from build123d import *

# Parameters (mm, degrees)
SKETCH_1_R      = 1.5
SKETCH_1_R_2    = 2
SKETCH_1_R_3    = 2.05
SKETCH_1_W      = 8.2
SKETCH_1_H      = 2.2
SKETCH_1_W_2    = 2.2
SKETCH_1_H_2    = 8.2
EXTRUDE_1_DEPTH = 2


with BuildPart() as part:
    # 草图1 → 凸台-拉伸1 (new body)
    with BuildSketch(Plane.XY):
        with BuildLine():
            Line((-51.22603831, 230.027402263), (-51.22603831, 124.402402263))
            Line((-51.22603831, 124.402402263), (-51.22603831, 0.652402263))
            Line((-51.22603831, 0.652402263), (-51.22603831, -5.881910062))
            Line((-51.22603831, -5.881910062), (-17.97603831, -5.881910062))
            Line((-17.97603831, -5.881910062), (19.52396169, -5.881910062))
            Line((19.52396169, -5.881910062), (52.77396169, -5.881910062))
            Line((52.77396169, -5.881910062), (52.77396169, 0.652402263))
            Line((52.77396169, 0.652402263), (52.77396169, 124.402402263))
            Line((52.77396169, 124.402402263), (52.77396169, 230.027402263))
            Line((52.77396169, 230.027402263), (33.77396169, 279.152402263))
            ThreePointArc((33.77396169, 279.152402263), (24.908633844, 301.658348145), (3.075925324, 312.072015922))
            Line((3.075925324, 312.072015922), (0.77396169, 314.152402263))
            Line((0.77396169, 314.152402263), (-1.528001943, 312.072015922))
            ThreePointArc((-1.528001943, 312.072015922), (-23.360710463, 301.658348145), (-32.22603831, 279.152402263))
            Line((-32.22603831, 279.152402263), (-51.22603831, 230.027402263))
        make_face()
        with Locations((-32.22603831, -0.347597737)):
            Circle(SKETCH_1_R, mode=Mode.SUBTRACT)
        with Locations((-48.22603831, 62.527402263)):
            Circle(SKETCH_1_R, mode=Mode.SUBTRACT)
        with Locations((-48.22603831, 186.277402263)):
            Circle(SKETCH_1_R, mode=Mode.SUBTRACT)
        with Locations((33.77396169, -0.347597737)):
            Circle(SKETCH_1_R, mode=Mode.SUBTRACT)
        with Locations((49.77396169, 62.527402263)):
            Circle(SKETCH_1_R, mode=Mode.SUBTRACT)
        with Locations((49.77396169, 186.277402263)):
            Circle(SKETCH_1_R, mode=Mode.SUBTRACT)
        with Locations((0.77396169, 21.118089938)):
            Circle(SKETCH_1_R, mode=Mode.SUBTRACT)
        with Locations((0.77396169, 31.118089938)):
            Circle(SKETCH_1_R, mode=Mode.SUBTRACT)
        with Locations((-14.22603831, 279.152402263)):
            Circle(SKETCH_1_R_2, mode=Mode.SUBTRACT)
        with Locations((-6.72603831, 292.14278332)):
            Circle(SKETCH_1_R_2, mode=Mode.SUBTRACT)
        with Locations((8.27396169, 292.14278332)):
            Circle(SKETCH_1_R_2, mode=Mode.SUBTRACT)
        with Locations((15.77396169, 279.152402263)):
            Circle(SKETCH_1_R_2, mode=Mode.SUBTRACT)
        with Locations((8.27396169, 266.162021207)):
            Circle(SKETCH_1_R_2, mode=Mode.SUBTRACT)
        with Locations((-6.72603831, 266.162021207)):
            Circle(SKETCH_1_R_2, mode=Mode.SUBTRACT)
        with Locations((0.77396169, 292.682402263)):
            Circle(SKETCH_1_R_3, mode=Mode.SUBTRACT)
        with Locations((12.491285404, 272.387402263)):
            Circle(SKETCH_1_R_3, mode=Mode.SUBTRACT)
        with Locations((-10.943362023, 272.387402263)):
            Circle(SKETCH_1_R_3, mode=Mode.SUBTRACT)
        with Locations((0.77396169, 246.152402263)):
            Circle(SKETCH_1_R, mode=Mode.SUBTRACT)
        with Locations((-16.97603831, -0.347597737)):
            Rectangle(SKETCH_1_W, SKETCH_1_H, mode=Mode.SUBTRACT)
        with Locations((18.52396169, -0.347597737)):
            Rectangle(SKETCH_1_W, SKETCH_1_H, mode=Mode.SUBTRACT)
        with BuildLine():
            Line((23.27396169, 191.554247886), (23.27396169, 61.554247886))
            ThreePointArc((23.27396169, 61.554247886), (0.77396169, 39.054247886), (-21.72603831, 61.554247886))
            Line((-21.72603831, 61.554247886), (-21.72603831, 191.554247886))
            ThreePointArc((-21.72603831, 191.554247886), (0.77396169, 214.054247886), (23.27396169, 191.554247886))
        make_face(mode=Mode.SUBTRACT)
        with Locations((-48.22603831, 217.714902263)):
            Rectangle(SKETCH_1_W_2, SKETCH_1_H_2, mode=Mode.SUBTRACT)
        with Locations((-48.22603831, 154.839902263)):
            Rectangle(SKETCH_1_W_2, SKETCH_1_H_2, mode=Mode.SUBTRACT)
        with Locations((-48.22603831, 93.964902263)):
            Rectangle(SKETCH_1_W_2, SKETCH_1_H_2, mode=Mode.SUBTRACT)
        with Locations((-48.22603831, 31.089902263)):
            Rectangle(SKETCH_1_W_2, SKETCH_1_H_2, mode=Mode.SUBTRACT)
        with Locations((49.77396169, 31.089902263)):
            Rectangle(SKETCH_1_W_2, SKETCH_1_H_2, mode=Mode.SUBTRACT)
        with Locations((49.77396169, 93.964902263)):
            Rectangle(SKETCH_1_W_2, SKETCH_1_H_2, mode=Mode.SUBTRACT)
        with Locations((49.77396169, 154.839902263)):
            Rectangle(SKETCH_1_W_2, SKETCH_1_H_2, mode=Mode.SUBTRACT)
        with Locations((49.77396169, 217.714902263)):
            Rectangle(SKETCH_1_W_2, SKETCH_1_H_2, mode=Mode.SUBTRACT)
        with Locations((0.77396169, 231.152402263)):
            Rectangle(SKETCH_1_W_2, SKETCH_1_H_2, mode=Mode.SUBTRACT)
        with Locations((0.77396169, 279.152402263)):
            Rectangle(SKETCH_1_W_2, SKETCH_1_H_2, mode=Mode.SUBTRACT)
    extrude(amount=EXTRUDE_1_DEPTH)


solid = part.part
Verification items for the finished model (mm, model axes). Round coordinates to 2 decimals unless told otherwise and drop trailing zeros. Order: outer loops, then holes, each group sorted by start corner. A loop starts at its lowest first (then second) coordinate and runs counter-clockwise, first axis right, second up. Notation, with made-up numbers: (-26.5, 77) -> (19.5, 77) arc R33 cw to (19.5, 107) -> close; hole circle Ø10 at (-11.75, -2). An arc over 180 degrees is marked (long way). Put each result on its own line as item: value.
1) Section check A-A (y = 178). Record the cut outline in (x, z), then the cut area to 3 significant figures.
Final values:
outline: (-51.23, 0) -> (-21.73, 0) -> (-21.73, 2) -> (-51.23, 2) -> close; (23.27, 0) -> (52.77, 0) -> (52.77, 2) -> (23.27, 2) -> close
area: 118 mm^2
2) Depth check by flat-ended pin: pin 1 (0.6 mm diameter, centred on x = -18, z = 1.5, fed in from +Y); pin 2 (3.5 mm diameter, centred on x = -14.23, y = 279.15, fed in from +Z); pin 3 (1 mm diameter, centred on y = 280, z = 1.5, fed in from +X). Enter the tip coordinate at first touch or a pass-through.
Final values:
pin 1: stops at y = 306.5
pin 2: passes through
pin 3: stops at x = 33.77
3) Section check D-D (y = 260.5). Record the cut outline in (x, z), then the cut area to 3 significant figures.
Final values:
outline: (-39.44, 0) -> (40.99, 0) -> (40.99, 2) -> (-39.44, 2) -> close
area: 161 mm^2
4) Mould release check, pull along X, two halves, no side actions. Record for faces 1 (the flat face through (-23, 156, 0)), 2 (the cylindrical face through (0.28, 214.05, 0.99)), 3 (the cylindrical face through (1.27, 39.06, 0.99)), 4 (the flat face through (43.407, 254.246, 0.986)): +X half, -X half, draft (parallel to the pull), parting line (faces both ways), or undercut.
Final values:
face 1: draft
face 2: undercut
face 3: undercut
face 4: +X half
5) Section check B-B (x = -41.5). Record the cut outline in (y, z), then the cut area to 3 significant figures.
Final values:
outline: (-5.88, 0) -> (255.17, 0) -> (255.17, 2) -> (-5.88, 2) -> close
area: 522 mm^2
6) Section check C-C (z = 1.65). Give the number of separate pieces and of enclosed holes in the cut face, then the cut area to 3 significant figures.
Final values:
separate pieces: 1
enclosed holes: 31
area: 22,600 mm^2
7) Material ranges on line 1 (X direction, y = 97, z = 1.65); line 2 (X direction, y = 33.5, z = 1.1); line 3 (X direction, y = 163, z = 1.45), recorded low to high.
Final values:
line 1: x = -51.23 to -49.33, -47.13 to -21.73, 23.27 to 48.67, 50.87 to 52.77
line 2: x = -51.23 to -49.33, -47.13 to 48.67, 50.87 to 52.77
line 3: x = -51.23 to -21.73, 23.27 to 52.77
